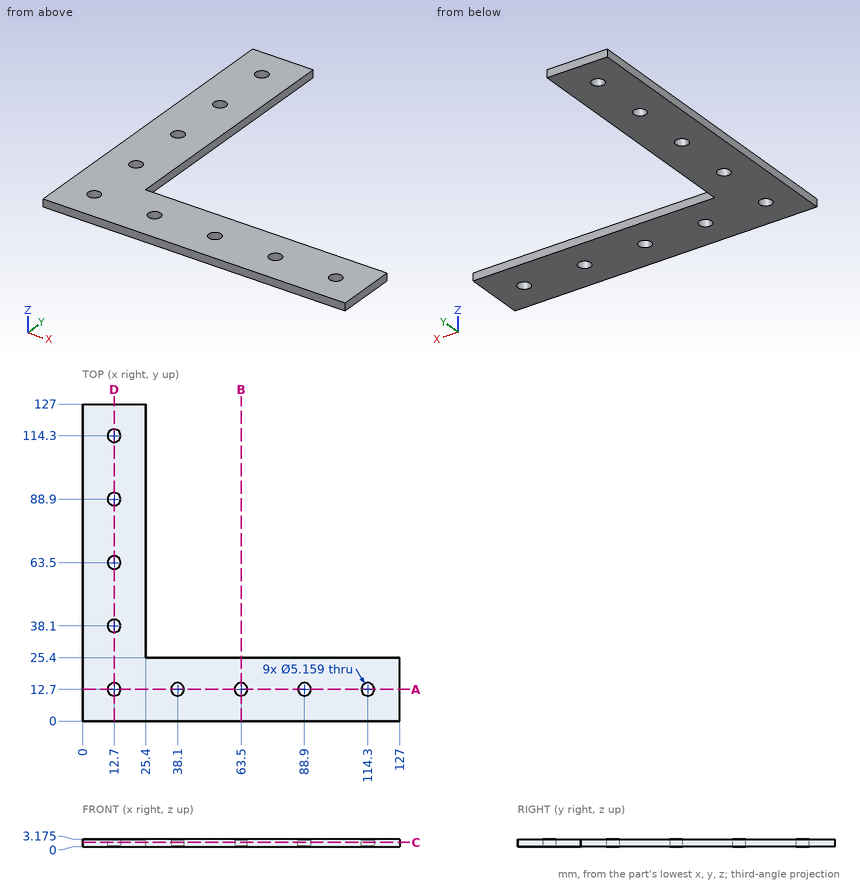
The drawing under review shows one solid part. Ordinate dimensions are in mm from its lowest x, y, z. Coordinates: 2 decimals unless noted, no trailing zeros. Order: outer loops, then holes, each group sorted by start corner. A loop starts at its lowest first (then second) coordinate and runs counter-clockwise, first axis right, second up. Notation, with made-up numbers: (-23, -2) -> (8, -2) arc R33 cw to (8, 33) -> close; hole circle Ø3 at (0, -34). An arc over 180 degrees is marked (long way). Answer in a Markdown table with one row per item. Add a question column.
Item 1: We need section A-A on y = 12.7. Write out the cut boundary in (x, z) (1 decimal).
Item 2: We need section C-C on z = 1.85. Give the number of separate pieces and of enclosed holes in the cut face, plus the area to 3 significant figures.
Item 3: Clearance check with flat-ended pins moving along their axes: pin 1 (6 mm diameter, centred on x = 12.7, y = 38.1, fed in from -Z); pin 2 (1.6 mm diameter, centred on y = 62, z = 1.5, fed in from +X); pin 3 (1 mm diameter, centred on x = 84.5, z = 1, fed in from +Y). State where each tip first meets the part, or that it passes through.
Item 4: To check wall thickness, follow probe 1 along Y at (x, z) = (12.7, 1.3); probe 2 along Y at (x, z) = (38.1, 0.9); probe 3 along X at (y, z) = (98, 2.35). State the ranges of each line that lie inside material, in increasing order.
Item 5: We need section B-B on x = 63.5. Write out the cut boundary in (y, z) (1 decimal).
Final values:
| question | item | result |
|---|---|---|
| 1 | outline | (0, 0) -> (10.1, 0) -> (10.1, 3.2) -> (0, 3.2) -> close; (15.3, 0) -> (35.5, 0) -> (35.5, 3.2) -> (15.3, 3.2) -> close; (40.7, 0) -> (60.9, 0) -> (60.9, 3.2) -> (40.7, 3.2) -> close; (66.1, 0) -> (86.3, 0) -> (86.3, 3.2) -> (66.1, 3.2) -> close; (91.5, 0) -> (111.7, 0) -> (111.7, 3.2) -> (91.5, 3.2) -> close; (116.9, 0) -> (127, 0) -> (127, 3.2) -> (116.9, 3.2) -> close |
| 2 | separate pieces | 1 |
| 2 | enclosed holes | 9 |
| 2 | area | 5,620 mm2 |
| 3 | pin 1 | stops at z = 0 |
| 3 | pin 2 | stops at x = 25.4 |
| 3 | pin 3 | stops at y = 25.4 |
| 4 | probe 1 | y = 0 to 10.12, 15.28 to 35.52, 40.68 to 60.92, 66.08 to 86.32, 91.48 to 111.72, 116.88 to 127 |
| 4 | probe 2 | y = 0 to 10.12, 15.28 to 25.4 |
| 4 | probe 3 | x = 0 to 25.4 |
| 5 | outline | (0, 0) -> (10.1, 0) -> (10.1, 3.2) -> (0, 3.2) -> close; (15.3, 0) -> (25.4, 0) -> (25.4, 3.2) -> (15.3, 3.2) -> close |
